Model file for the job. Use its own axes, mm. A direction names the side the tool comes from. Round coordinates to 2 decimals unless told otherwise and drop trailing zeros. Loops run counter-clockwise (first coordinate to the right, second up) from the corner with the lowest first, then second, coordinate; pieces in that order, holes last. Notation, with made-up numbers: M 46.25,33.25 L 96.25,33.25 A13 ccw 96.25,56.25 Z; hole C -9,44 d4. An arc over 180 degrees is marked long. Use a Markdown table: item, result. Add a question column.
Item 1: Saw through at B-B on z = -6.5. Write the cut outline in (x, y) (1 decimal), then the cut area to 3 significant figures.
Item 2: Saw through at C-C on x = 19. Write the cut outline in (y, z) (1 decimal), then the cut area to 3 significant figures.
Item 3: Pin check, flat tips, straight feed: P1, Ø1, axis at x = 15.5, y = 63, coming from the +Z side; P2, Ø4, axis at x = -23.5, z = -2, coming from the -Y side; P3, Ø5, axis at y = 32, z = 8.5, coming from the +X side; P4, Ø10, axis at x = 25.5, y = 26, coming from the -Z side. Stop position of each tip, or through.
Item 4: Tool access for faces 1 (the flat face through (-16, 12.7, -24)), 2 (the flat face through (17, 71.438, -15)): list every direction of +Z, -Z, +X, -X, +Y, -Y with a clear straight run to the whole face (end or side of a thin tool).
Item 5: Saw through at A-A on x = 0. Write the cut outline in (y, z) (1 decimal).
Item 6: Saw through at D-D on z = -18.5. Write the cut outline in (x, y) (1 decimal), then the cut area to 3 significant figures.
Item 7: Wall check: L1, parallel to X at y = 70.65, z = 0 (3 decimals); L2, parallel to X at y = 11.5, z = -30; L3, parallel to X at y = 11.5, z = -27 (3 decimals). Give the ranges that are in metal, low to high. Write a range as from..to.
Item 8: Two-plate mould, pull along Z, no slides. Class faces 3 (the flat face through (-34.925, 6, 0)), 4 (the cylindrical face through (-1.256, 41.658, 28.547)), 5 (the cylindrical face through (18.74, 69.87, 11.95)), 6 (the cylindrical face through (-30.727, 6.439, -27.203)): +Z half, -Z half, draft (parallel to the pull), parting line (faces both ways), or undercut.
```python
from build123d import *

# Parameters (mm, degrees)
SKETCH1_W           = 69.85
SKETCH1_H           = 69.85
BASE_EXTRUDE_DEPTH  = 12.7
SKETCH2_R           = 28.575
BOSS_EXTRUDE1_DEPTH = 71.4375
SKETCH3_R           = 12.7
CUT_EXTRUDE1_DEPTH  = 87.849453978
SKETCH4_R           = 22.225
CUT_EXTRUDE2_DEPTH  = 3.175
FILLET1_R           = 6.35
CIRPATTERN2_COUNT   = 4


with BuildPart() as part:
    # Sketch1 → Base-Extrude (new body)
    with BuildSketch(Plane(origin=(0, 0, 0), x_dir=(1, 0, 0), z_dir=(0, 1, 0))):
        Rectangle(SKETCH1_W, SKETCH1_H)
    extrude(amount=BASE_EXTRUDE_DEPTH)

    # Sketch2 → Boss-Extrude1 (add)
    with BuildSketch(Plane(origin=(0, 0, 0), x_dir=(-1, 0, 0), z_dir=(0, 1, 0))):
        with Locations(Location((0, 0, 0), (0, 0, 270))):
            Circle(SKETCH2_R)
    extrude(amount=BOSS_EXTRUDE1_DEPTH)

    # Sketch3 → Cut-Extrude1 (cut, through all)
    with BuildSketch(Plane(origin=(0, 71.4375, 0), x_dir=(-1, 0, 0), z_dir=(0, 1, 0))):
        with Locations(Location((0, 0, 0), (0, 0, 90))):
            Circle(SKETCH3_R)
    extrude(amount=-CUT_EXTRUDE1_DEPTH, mode=Mode.SUBTRACT)

    # Sketch4 → Cut-Extrude2 (cut)
    with BuildSketch(Plane(origin=(0, 71.4375, 0), x_dir=(-1, 0, 0), z_dir=(0, 1, 0))):
        with Locations(Location((0, 0, 0), (0, 0, 90))):
            Circle(SKETCH4_R)
    extrude(amount=-CUT_EXTRUDE2_DEPTH, mode=Mode.SUBTRACT)

    # Fillet1
    fillet1_edges = [part.edges().sort_by_distance(p)[0] for p in [
        (-34.925, 6.35, 34.925),
        (34.925, 6.35, 34.925),
        (34.925, 6.35, -34.925),
        (-34.925, 6.35, -34.925),
    ]]
    fillet(fillet1_edges, radius=FILLET1_R)

    # Sketch7 → 1/4-20 Tapped Hole2 (revolve, cut)
    with BuildSketch(Plane(origin=(-28.575, 12.7, -28.575), x_dir=(0, 0, 1), z_dir=(1, 0, 0))):
        Polygon((0, 0), (0, 20.583816902), (2.5527, 19.05), (2.5527, 0), align=None)
    f_1_4_20_tapped_hole2 = revolve(axis=Axis((-28.575, 19.05, -28.575), (0, -1, 0)), mode=Mode.SUBTRACT)

    # CirPattern2: 1/4-20 Tapped Hole2 ×4 about axis
    cirpattern2_axis = Axis((0, 0, 0), (0, 1, 0))
    for i in range(1, CIRPATTERN2_COUNT):
        add(f_1_4_20_tapped_hole2.rotate(cirpattern2_axis, i * 360 / CIRPATTERN2_COUNT), mode=Mode.SUBTRACT)


solid = part.part
```
Entries:
| question | item | result |
|---|---|---|
| 1 | outline | M -34.9,0 L -10.9,0 L -10.9,68.3 L -21.3,68.3 L -21.3,71.4 L -27.8,71.4 L -27.8,12.7 L -34.9,12.7 Z; M 10.9,0 L 34.9,0 L 34.9,12.7 L 27.8,12.7 L 27.8,71.4 L 21.3,71.4 L 21.3,68.3 L 10.9,68.3 Z |
| 1 | area | 2,530 mm2 |
| 2 | outline | M 0,-34.9 L 12.7,-34.9 L 12.7,-21.3 L 71.4,-21.3 L 71.4,-11.5 L 68.3,-11.5 L 68.3,11.5 L 71.4,11.5 L 71.4,21.3 L 12.7,21.3 L 12.7,34.9 L 0,34.9 Z |
| 2 | area | 3,320 mm2 |
| 3 | P1 | z = 24.32 |
| 3 | P2 | y = 0 |
| 3 | P3 | x = 27.94 |
| 3 | P4 | z = -19.91 |
| 4 | face 1 | +Y |
| 4 | face 2 | +Z, -Z, +X, -X, +Y |
| 5 | outline | M 0,-34.9 L 12.7,-34.9 L 12.7,-28.6 L 71.4,-28.6 L 71.4,-22.2 L 68.3,-22.2 L 68.3,-12.7 L 0,-12.7 Z; M 0,12.7 L 68.3,12.7 L 68.3,22.2 L 71.4,22.2 L 71.4,28.6 L 12.7,28.6 L 12.7,34.9 L 0,34.9 Z |
| 6 | outline | M -34.9,0 L 34.9,0 L 34.9,12.7 L 21.8,12.7 L 21.8,71.4 L 12.3,71.4 L 12.3,68.3 L -12.3,68.3 L -12.3,71.4 L -21.8,71.4 L -21.8,12.7 L -34.9,12.7 Z |
| 6 | area | 3,370 mm2 |
| 7 | L1 | -28.575..-22.225, 22.225..28.575 |
| 7 | L2 | -34.76..-30.69, -26.46..26.46, 30.69..34.76 |
| 7 | L3 | -34.925..-30.584, -26.566..26.566, 30.584..34.925 |
| 8 | face 3 | draft |
| 8 | face 4 | parting line |
| 8 | face 5 | undercut |
| 8 | face 6 | undercut |
